from build123d import *

# Parameters (mm, degrees)
BOSS_EXTRUDE1_OUTLINE_R = 1.75
BOSS_EXTRUDE1_DEPTH     = 4
CUT_EXTRUDE1_DEPTH      = 1


# Read off the part's stored shape, not the designer's step: Boss-Extrude1
with BuildPart() as part:
    # Boss-Extrude1 outline → Boss-Extrude1 (new body)
    with BuildSketch(Plane(origin=(0, 0, 0), x_dir=(1, 0, 0), z_dir=(0, 1, 0))):
        with BuildLine():
            Line((25.306474615, -10.33744254), (36.91307775, -10.33744254))
            ThreePointArc((36.91307775, -10.33744254), (39.349776183, -5.587442326), (41.786474615, -10.33744254))
            Line((41.786474615, -10.33744254), (48.849776182, -10.33744254))
            Line((48.849776182, -10.33744254), (48.849776182, -18.81631662))
            Line((48.849776182, -18.81631662), (58.749776182, -18.81631662))
            Line((58.749776182, -18.81631662), (58.749776182, -4.977921711))
            Line((58.749776182, -4.977921711), (-21.250223818, -4.977921711))
            Line((-21.250223818, -4.977921711), (-21.250223818, -18.81631662))
            Line((-21.250223818, -18.81631662), (-11.350223818, -18.81631662))
            Line((-11.350223818, -18.81631662), (-11.350223818, -10.33744254))
            Line((-11.350223818, -10.33744254), (3.95307775, -10.33744254))
            ThreePointArc((3.95307775, -10.33744254), (6.389776182, -5.587442326), (8.826474615, -10.33744254))
            Line((8.826474615, -10.33744254), (20.43307775, -10.33744254))
            ThreePointArc((20.43307775, -10.33744254), (22.869776182, -5.587442326), (25.306474615, -10.33744254))
        make_face()
        with Locations((-16.250223818, -13.587442433)):
            Circle(BOSS_EXTRUDE1_OUTLINE_R, mode=Mode.SUBTRACT)
        with Locations((53.749776182, -13.587442433)):
            Circle(BOSS_EXTRUDE1_OUTLINE_R, mode=Mode.SUBTRACT)
    extrude(amount=BOSS_EXTRUDE1_DEPTH)

    # Sketch2 → Cut-Extrude1 (cut)
    # profile 1 of 2: a face of its own
    with BuildSketch(Plane(origin=(0, 4, 0), x_dir=(1, 0, 0), z_dir=(0, 1, 0))):
        Polygon((-16.41198232, -6.812466594), (-14.865187448, -6.812466594), (-14.865187448, -7.382338389), (-15.842110525, -7.382338389), (-15.842110525, -7.992915312), (-14.865187448, -7.992915312), (-14.865187448, -8.562787107), (-15.842110525, -8.562787107), (-15.842110525, -9.987466594), (-16.41198232, -9.987466594), align=None)
    # profile 2 of 2: a face of its own
    with BuildSketch(Plane(origin=(0, 4, 0), x_dir=(1, 0, 0), z_dir=(0, 1, 0))):
        with BuildLine():
            add(Edge.make_bspline(
                [(-12.817210686, -8.277851209), (-12.783916812, -8.301640582), (-12.718014592, -8.348729498), (-12.630981866, -8.433091053), (-12.556016347, -8.527197346), (-12.493905254, -8.630471147), (-12.44414372, -8.740373961), (-12.408522012, -8.855731057), (-12.385895512, -8.975524957), (-12.383424023, -9.057083985), (-12.382174628, -9.09831395)],
                knots=[0, 0, 0, 0, 1.013736912, 2.006600758, 2.994453809, 3.989973287, 4.987781207, 5.978959008, 6.978317308, 8, 8, 8, 8], degree=3))
            add(Edge.make_bspline(
                [(-12.382174628, -9.09831395), (-12.383681928, -9.142958744), (-12.386671463, -9.231505963), (-12.413102949, -9.361360446), (-12.455537639, -9.486113154), (-12.513532925, -9.604387133), (-12.586248347, -9.71250688), (-12.671004934, -9.808223668), (-12.767909528, -9.889037688), (-12.858130451, -9.94386948), (-12.93578675, -9.980293202), (-12.998454703, -10.003603653), (-13.064627941, -10.024125244), (-13.134778669, -10.040520633), (-13.208894129, -10.053319925), (-13.28686855, -10.061772553), (-13.368753261, -10.067917099), (-13.424595172, -10.068551539), (-13.453228314, -10.06887685)],
                knots=[0, 0, 0, 0, 1.313679292, 2.605514271, 3.884962679, 5.186178731, 6.472827995, 7.711026938, 8.938935107, 10.174644318, 10.808706728, 11.462743532, 12.142127587, 12.847854939, 13.582806024, 14.355735269, 15.156897313, 16, 16, 16, 16], degree=3))
            add(Edge.make_bspline(
                [(-13.453228314, -10.06887685), (-13.483762719, -10.068462664), (-13.543390392, -10.067653841), (-13.630433512, -10.062763265), (-13.712540889, -10.05374694), (-13.789884756, -10.041877645), (-13.862390702, -10.026171129), (-13.930060872, -10.006256127), (-13.993058665, -9.983580681), (-14.070171273, -9.949055369), (-14.158297, -9.895136701), (-14.253544974, -9.816174366), (-14.337148326, -9.722127758), (-14.409833523, -9.615636751), (-14.467126735, -9.497356478), (-14.509731675, -9.370999371), (-14.534962825, -9.236907843), (-14.538000373, -9.145061739), (-14.539546423, -9.09831395)],
                knots=[0, 0, 0, 0, 0.886964665, 1.7320671, 2.531131818, 3.285397207, 4.004107883, 4.684213108, 5.332925796, 5.947568694, 7.135706876, 8.320776993, 9.52873045, 10.778999824, 12.05415135, 13.333578234, 14.642845846, 16, 16, 16, 16], degree=3))
            add(Edge.make_bspline(
                [(-14.539546423, -9.09831395), (-14.538133592, -9.057534194), (-14.535357209, -8.977397037), (-14.515469601, -8.859970757), (-14.481368397, -8.74863675), (-14.434576238, -8.642619953), (-14.374238543, -8.54190857), (-14.29999851, -8.447243639), (-14.212797428, -8.357771149), (-14.146671217, -8.304933073), (-14.112778594, -8.277851209)],
                knots=[0, 0, 0, 0, 1.01821053, 2.000906977, 2.963938143, 3.919209931, 4.888045165, 5.887808425, 6.917407893, 8, 8, 8, 8], degree=3))
            add(Edge.make_bspline(
                [(-14.112778594, -8.277851209), (-14.133790223, -8.25361737), (-14.175155792, -8.205908238), (-14.228683245, -8.129124193), (-14.27377787, -8.049959762), (-14.312065354, -7.969057406), (-14.340368438, -7.885024188), (-14.361772094, -7.799181284), (-14.373877981, -7.710654149), (-14.375770168, -7.650984229), (-14.37672591, -7.620844999)],
                knots=[0, 0, 0, 0, 1.061529281, 2.089831458, 3.092927091, 4.075998741, 5.048384512, 6.024008542, 7.00192825, 8, 8, 8, 8], degree=3))
            add(Edge.make_bspline(
                [(-14.37672591, -7.620844999), (-14.375458741, -7.580045367), (-14.372958667, -7.499549264), (-14.35081565, -7.381844957), (-14.314052865, -7.270002405), (-14.264040225, -7.164349068), (-14.200531945, -7.067187545), (-14.125070359, -6.98005538), (-14.036594626, -6.906144188), (-13.93839492, -6.842725124), (-13.829979018, -6.792282188), (-13.71237556, -6.756985999), (-13.587004623, -6.734641651), (-13.500602716, -6.732269623), (-13.456408402, -6.731056337)],
                knots=[0, 0, 0, 0, 1.022455555, 2.017265428, 2.990720743, 3.968117071, 4.939886797, 5.893155559, 6.847550415, 7.820889576, 8.817530429, 9.83499769, 10.892607882, 12, 12, 12, 12], degree=3))
            add(Edge.make_bspline(
                [(-13.456408402, -6.731056337), (-13.412850602, -6.732271608), (-13.327922012, -6.734641132), (-13.204754302, -6.756837427), (-13.089692277, -6.792919844), (-12.983687415, -6.844427856), (-12.886503285, -6.907969153), (-12.799531264, -6.984453863), (-12.724306479, -7.073756197), (-12.66027104, -7.173431259), (-12.609244635, -7.280816697), (-12.571520994, -7.393432622), (-12.549701195, -7.510393862), (-12.546570098, -7.589805025), (-12.544995141, -7.629749246)],
                knots=[0, 0, 0, 0, 1.094655142, 2.134348324, 3.136019022, 4.118575226, 5.088726318, 6.048298823, 7.020513804, 8.015920439, 9.020015034, 10.003048569, 10.995523219, 12, 12, 12, 12], degree=3))
            add(Edge.make_bspline(
                [(-12.544995141, -7.629749246), (-12.545753836, -7.657979661), (-12.547242718, -7.713379741), (-12.558251211, -7.794999693), (-12.576788162, -7.873314147), (-12.60263287, -7.950215641), (-12.638565836, -8.027794016), (-12.687191493, -8.107535817), (-12.746338221, -8.19275433), (-12.792789101, -8.248528105), (-12.817210686, -8.277851209)],
                knots=[0, 0, 0, 0, 0.940746401, 1.846144481, 2.739104268, 3.619506754, 4.545839139, 5.581956076, 6.728711598, 8, 8, 8, 8], degree=3))
        make_face()
        with BuildLine():
            add(Edge.make_bspline(
                [(-13.47040079, -7.300928132), (-13.493863602, -7.302059257), (-13.539503955, -7.304259544), (-13.604627394, -7.324119575), (-13.66317549, -7.356602067), (-13.713811769, -7.401304369), (-13.755336157, -7.455543915), (-13.7858543, -7.517903357), (-13.80395192, -7.58761311), (-13.805867905, -7.6364252), (-13.806854115, -7.661550128)],
                knots=[0, 0, 0, 0, 1.018099191, 1.980427864, 2.929421084, 3.909248076, 4.895556904, 5.880788387, 6.909183412, 8, 8, 8, 8], degree=3))
            add(Edge.make_bspline(
                [(-13.806854115, -7.661550128), (-13.805635844, -7.686889627), (-13.803257052, -7.736367441), (-13.784550526, -7.807416545), (-13.752664735, -7.871807238), (-13.70888576, -7.92819461), (-13.655687215, -7.974250185), (-13.596121153, -8.00942487), (-13.529526976, -8.029505185), (-13.483250413, -8.032228147), (-13.45958849, -8.03362044)],
                knots=[0, 0, 0, 0, 1.07118507, 2.091592095, 3.082435519, 4.092579768, 5.090825648, 6.043203473, 6.999459622, 8, 8, 8, 8], degree=3))
            add(Edge.make_bspline(
                [(-13.45958849, -8.03362044), (-13.435479226, -8.032541652), (-13.388509856, -8.03043997), (-13.321749401, -8.009838627), (-13.261606764, -7.976890976), (-13.21010348, -7.930310288), (-13.16744294, -7.873902495), (-13.136374254, -7.808386518), (-13.118492241, -7.734993318), (-13.116104929, -7.683698208), (-13.114866936, -7.657098004)],
                knots=[0, 0, 0, 0, 1.008803858, 1.965339183, 2.900766489, 3.864508618, 4.855158575, 5.849593072, 6.884859315, 8, 8, 8, 8], degree=3))
            add(Edge.make_bspline(
                [(-13.114866936, -7.657098004), (-13.116136245, -7.631989686), (-13.118591044, -7.583431082), (-13.136192895, -7.513716807), (-13.168519575, -7.452330647), (-13.210992661, -7.398427917), (-13.264242529, -7.354958718), (-13.326061725, -7.322991206), (-13.395995039, -7.304449741), (-13.445061785, -7.302127422), (-13.47040079, -7.300928132)],
                knots=[0, 0, 0, 0, 1.065910571, 2.061433587, 3.023559535, 3.990682701, 4.956464619, 5.918590567, 6.925120432, 8, 8, 8, 8], degree=3))
        make_face(mode=Mode.SUBTRACT)
        with BuildLine():
            add(Edge.make_bspline(
                [(-13.451956279, -8.603492235), (-13.46978624, -8.603788328), (-13.50492887, -8.604371924), (-13.556591424, -8.611101658), (-13.606166954, -8.621130626), (-13.653593954, -8.634965304), (-13.698632825, -8.653825453), (-13.741665347, -8.67656171), (-13.782542906, -8.703403911), (-13.820659173, -8.733864736), (-13.855107371, -8.767298393), (-13.886159288, -8.802168614), (-13.911539847, -8.839376887), (-13.9326758, -8.8776864), (-13.949658659, -8.917400732), (-13.960885612, -8.959173898), (-13.968114198, -9.002449596), (-13.969151425, -9.031927247), (-13.969674628, -9.046796522)],
                knots=[0, 0, 0, 0, 1.129580664, 2.226389355, 3.296443603, 4.333934503, 5.352185725, 6.386189251, 7.41493955, 8.447544828, 9.47401038, 10.455044306, 11.4018853, 12.322125673, 13.225630306, 14.132028716, 15.057747923, 16, 16, 16, 16], degree=3))
            add(Edge.make_bspline(
                [(-13.969674628, -9.046796522), (-13.96942526, -9.062303707), (-13.968930669, -9.09306029), (-13.961460572, -9.137952007), (-13.950704952, -9.181246985), (-13.93559834, -9.222539958), (-13.915396116, -9.261806883), (-13.891274294, -9.299429521), (-13.862391756, -9.335144056), (-13.829531642, -9.368758999), (-13.79274489, -9.399085677), (-13.753096834, -9.425804009), (-13.711111133, -9.449360258), (-13.665527406, -9.466326402), (-13.618033802, -9.481855308), (-13.56735795, -9.491276321), (-13.514053346, -9.498208564), (-13.47763421, -9.498735008), (-13.458952473, -9.499005055)],
                knots=[0, 0, 0, 0, 0.973817353, 1.931446211, 2.852767904, 3.776304432, 4.688323523, 5.623710549, 6.581246645, 7.570897993, 8.57436511, 9.572506873, 10.574556662, 11.591826551, 12.624694332, 13.712108235, 14.826391851, 16, 16, 16, 16], degree=3))
            add(Edge.make_bspline(
                [(-13.458952473, -9.499005055), (-13.440068015, -9.498662752), (-13.403268187, -9.497995712), (-13.349474239, -9.492100337), (-13.298594712, -9.482746092), (-13.250690378, -9.469367342), (-13.205580086, -9.452228631), (-13.163868953, -9.430414443), (-13.124604643, -9.405692898), (-13.089048919, -9.37681074), (-13.056583922, -9.345335216), (-13.02861077, -9.310840719), (-13.004825508, -9.274436466), (-12.985640103, -9.235729111), (-12.970159203, -9.194901366), (-12.959540278, -9.151546137), (-12.952950853, -9.106150636), (-12.952351136, -9.075228349), (-12.952046423, -9.059516874)],
                knots=[0, 0, 0, 0, 1.200705402, 2.339794563, 3.437264955, 4.487414319, 5.499029866, 6.500076882, 7.476298407, 8.444948224, 9.407950986, 10.347155707, 11.263432813, 12.167927724, 13.089546445, 14.03463663, 15.00140776, 16, 16, 16, 16], degree=3))
            add(Edge.make_bspline(
                [(-12.952046423, -9.059516874), (-12.952628246, -9.043599995), (-12.953765508, -9.012488012), (-12.959988437, -8.966543851), (-12.971662018, -8.922988069), (-12.986934472, -8.880810497), (-13.007250343, -8.840883929), (-13.032472057, -8.80329263), (-13.061180558, -8.767105421), (-13.094734453, -8.733933223), (-13.131420419, -8.703602043), (-13.170466782, -8.676580291), (-13.211753276, -8.65369536), (-13.255392832, -8.634988065), (-13.301544899, -8.621123427), (-13.349857336, -8.61110201), (-13.40025089, -8.604370418), (-13.434549713, -8.603787874), (-13.451956279, -8.603492235)],
                knots=[0, 0, 0, 0, 1.011708178, 1.977538892, 2.938094892, 3.871441737, 4.823268678, 5.775953079, 6.743660653, 7.753304209, 8.767430709, 9.76505158, 10.765940967, 11.761741361, 12.775867861, 13.822051386, 14.89469657, 16, 16, 16, 16], degree=3))
        make_face(mode=Mode.SUBTRACT)
    extrude(amount=-CUT_EXTRUDE1_DEPTH, mode=Mode.SUBTRACT)


solid = part.part
Check sheet for the modelled part. Datum: model origin and axes. Units: mm. A direction names the side the tool comes from. Give positions to 0.01 mm unless a question says otherwise; leave off trailing zeros. Write each loop counter-clockwise with the first axis right and the second up, starting at its lowest first coordinate (ties: lowest second). Pieces come first, ordered by that corner, then holes. Notation, with made-up numbers: (89.5, -23) -> (142.5, -23) arc R15 ccw to (142.5, -9) -> close; hole circle Ø1 at (-37.5, 47.5). An arc over 180 degrees is marked (long way). One line per item, written item: value. Start each with the question number.
Item 1: Gauge pin test, flat ends, axial feed: pin 1 (7 mm diameter, centred on x = 39.35, z = 8.59, fed in from -Y); pin 2 (2 mm diameter, centred on x = 29.5, y = 1, fed in from +Z). Record the tip position at first contact, or that the pin passes through.
Item 2: Draft check along X on faces 1 (the flat face through (-21.25, 2, 12)), 2 (the cylindrical face through (6.3, 1.97, 5.59)), 3 (the flat face through (18, 0, 9)). Enter one of: +X half, -X half, draft (parallel to the pull), parting line (faces both ways), or undercut.
Item 3: Section check B-B on y = 1.4. Record the cut outline in (x, z), then the cut area to 3 significant figures.
Item 4: Material ranges on probe 1 along X at (y, z) = (0.45, 18.25); probe 2 along X at (y, z) = (1, 7.5); probe 3 along X at (y, z) = (2.15, 14.75), recorded low to high. Write a range as from..to.
Item 5: Section check C-C on x = 46.5. Record the cut outline in (y, z).
Item 6: Tool access check on faces 4 (the flat face through (-13, 3, 8)), 5 (the flat face through (54, 2, 18.816)), 6 (the flat face through (-4, 2, 10.337)). Record the directions out of +Z, -Z, +X, -X, +Y, -Y that give a thin tool (end or side, any length) a straight path to the whole face; none if there is none.
Item 7: Section check A-A on z = 16. Record the cut outline in (x, y).
Item 8: Section check D-D on x = 8. Record the cut outline in (y, z).
Results list:
1. pin 1: y = 0
1. pin 2: z = 10.34
2. face 1: -X half
2. face 2: undercut
2. face 3: draft
3. outline: (-21.25, 4.98) -> (58.75, 4.98) -> (58.75, 18.82) -> (48.85, 18.82) -> (48.85, 10.34) -> (41.79, 10.34) arc R3 cw (long way) to (36.91, 10.34) -> (25.31, 10.34) arc R3 cw (long way) to (20.43, 10.34) -> (8.83, 10.34) arc R3 cw (long way) to (3.95, 10.34) -> (-11.35, 10.34) -> (-11.35, 18.82) -> (-21.25, 18.82) -> close; hole circle Ø3.5 at (-16.25, 13.59); hole circle Ø3.5 at (53.75, 13.59)
3. area: 505 mm²
4. probe 1: -21.25..-11.35, 48.85..58.75
4. probe 2: -21.25..3.59, 9.19..20.07, 25.67..36.55, 42.15..58.75
4. probe 3: -21.25..-17.56, -14.94..-11.35, 48.85..52.44, 55.06..58.75
5. outline: (0, 4.98) -> (4, 4.98) -> (4, 10.34) -> (0, 10.34) -> close
6. face 4: +Y
6. face 5: +Z, +X, -X, +Y, -Y
6. face 6: +Z, +Y, -Y
7. outline: (-21.25, 0) -> (-11.35, 0) -> (-11.35, 4) -> (-21.25, 4) -> close; (48.85, 0) -> (58.75, 0) -> (58.75, 4) -> (48.85, 4) -> close
8. outline: (0, 4.98) -> (4, 4.98) -> (4, 6.06) -> (0, 6.06) -> close
